Source: CAD feature listing. Evaluate the final solid. Frame: model axes, mm. Give positions to 0.01 mm unless a question says otherwise; leave off trailing zeros. Loops run counter-clockwise (first coordinate to the right, second up) from the corner with the lowest first, then second, coordinate; pieces in that order, holes last. Notation, with made-up numbers: M -27,73.5 L -8,73.5 A22 cw -8,87.5 Z; hole C 14,4 d6. An arc over 180 degrees is marked long. Answer in a Markdown table with one row per item.
```python
from build123d import *

# Parameters (mm, degrees)
EXTRUDE_1_DEPTH     = 3
EXTRUDE_2_DEPTH     = 200
FILLET_1_R          = 4
SKETCH_4_W          = 25
SKETCH_4_H          = 25
CUT_EXTRUDE_1_DEPTH = 4
FILLET_3_R          = 8
SKETCH_5_W          = 15
SKETCH_5_H          = 20
CUT_EXTRUDE_2_DEPTH = 10
FILLET_4_R          = 10
FILLET_5_R          = 10
SKETCH_7_R          = 1.05
SKETCH_7_R_2        = 1
CUT_EXTRUDE_3_DEPTH = 5


with BuildPart() as part:
    # 草图1 → 凸台-拉伸1 (new body)
    with BuildSketch(Plane.XY):
        Polygon((-68.534318099, 4.283164377), (-80.94435421, -20.816457208), (-55.844732625, -33.22649332), (-43.434696514, -8.126871734), align=None)
    extrude(amount=EXTRUDE_1_DEPTH)

    # 草图2 → 凸台-拉伸2 (add)
    with BuildSketch(Plane.XY.offset(3)):
        Polygon((-87.038364402, -64.656684429), (-38.284651107, 33.948971798), (-35.595405937, 32.619325071), (-84.349119232, -65.986331156), align=None)
    extrude(amount=EXTRUDE_2_DEPTH)

    # 圆角1
    fillet_1_edges = [part.edges().sort_by_distance(p)[0] for p in [
        (-59.529047009, -15.787087985, 3),
        (-62.218292179, -14.457441259, 3),
    ]]
    fillet(fillet_1_edges, radius=FILLET_1_R)

    # 草图4 → 切除-拉伸1 (cut)
    with BuildSketch(Plane(origin=(-44.25211262, 21.879625307, 0), x_dir=(0, 0, 1), z_dir=(-0.8964150566080468, 0.4432155754104229, 0))):
        with Locations((15.5, -84.035984194)):
            Rectangle(SKETCH_4_W, SKETCH_4_H)
    extrude(amount=-CUT_EXTRUDE_1_DEPTH, mode=Mode.SUBTRACT)

    # 圆角3
    fillet_3_edges = [part.edges().sort_by_distance(p)[0] for p in [
        (-74.613352432, -42.911131377, 3),
        (-74.613352432, -42.911131377, 28),
    ]]
    fillet(fillet_3_edges, radius=FILLET_3_R)

    # 草图5 → 切除-拉伸2 (cut)
    with BuildSketch(Plane(origin=(-41.56286745, 20.54997858, 0), x_dir=(0, 0, -1), z_dir=(0.8964150566080469, -0.4432155754104229, 0))):
        with Locations((-60.5, -11.535984194)):
            Rectangle(SKETCH_5_W, SKETCH_5_H)
        with Locations((-30.5, -11.535984194)):
            Rectangle(SKETCH_5_W, SKETCH_5_H)
        with Locations((-90.5, -11.535984194)):
            Rectangle(SKETCH_5_W, SKETCH_5_H)
        with Locations((-120.5, -11.535984194)):
            Rectangle(SKETCH_5_W, SKETCH_5_H)
        with Locations((-150.5, -11.535984194)):
            Rectangle(SKETCH_5_W, SKETCH_5_H)
        with Locations((-180.5, -11.535984194)):
            Rectangle(SKETCH_5_W, SKETCH_5_H)
        with Locations((-60.5, -41.535984194)):
            Rectangle(SKETCH_5_W, SKETCH_5_H)
        with Locations((-90.5, -41.535984194)):
            Rectangle(SKETCH_5_W, SKETCH_5_H)
        with Locations((-120.5, -41.535984194)):
            Rectangle(SKETCH_5_W, SKETCH_5_H)
        with Locations((-150.5, -41.535984194)):
            Rectangle(SKETCH_5_W, SKETCH_5_H)
        with Locations((-180.5, -41.535984194)):
            Rectangle(SKETCH_5_W, SKETCH_5_H)
        with Locations((-60.5, -71.535984194)):
            Rectangle(SKETCH_5_W, SKETCH_5_H)
        with Locations((-90.5, -71.535984194)):
            Rectangle(SKETCH_5_W, SKETCH_5_H)
        with Locations((-120.5, -71.535984194)):
            Rectangle(SKETCH_5_W, SKETCH_5_H)
        with Locations((-150.5, -71.535984194)):
            Rectangle(SKETCH_5_W, SKETCH_5_H)
        with Locations((-180.5, -71.535984194)):
            Rectangle(SKETCH_5_W, SKETCH_5_H)
        with Locations((-30.5, -41.535984194)):
            Rectangle(SKETCH_5_W, SKETCH_5_H)
    extrude(amount=-CUT_EXTRUDE_2_DEPTH, mode=Mode.SUBTRACT)

    # 圆角4
    fillet_4_edges = [part.edges().sort_by_distance(p)[0] for p in [
        (-36.940028522, 33.284148434, 203),
    ]]
    fillet(fillet_4_edges, radius=FILLET_4_R)

    # 圆角5
    fillet_5_edges = [part.edges().sort_by_distance(p)[0] for p in [
        (-36.940028522, 33.284148434, 3),
    ]]
    fillet(fillet_5_edges, radius=FILLET_5_R)

    # 草图7 → 切除-拉伸3 (cut)
    with BuildSketch(Plane(origin=(0, 0, 0), x_dir=(-1, 0, 0), z_dir=(0, 0, -1))):
        with Locations((48.793219042, -9.939669659)):
            Circle(SKETCH_7_R)
        with Locations((66.721520174, -1.075358151)):
            Circle(SKETCH_7_R)
        with Locations((71.153675928, -10.039508717)):
            Circle(SKETCH_7_R_2)
        with Locations((68.912638286, -11.147547656)):
            Circle(SKETCH_7_R_2)
        with Locations((75.585831682, -19.003659283)):
            Circle(SKETCH_7_R)
        with Locations((57.65753055, -27.867970791)):
            Circle(SKETCH_7_R)
        with Locations((53.225374796, -18.903820225)):
            Circle(SKETCH_7_R_2)
        with Locations((55.466412437, -17.795781287)):
            Circle(SKETCH_7_R_2)
    extrude(amount=-CUT_EXTRUDE_3_DEPTH, mode=Mode.SUBTRACT)


solid = part.part
```
1) Material intervals for L1, parallel to Z at x = -79.5, y = -21; L2, parallel to Y at x = -71, z = 127; L3, parallel to X at y = -17.5, z = 74, sorted ascending.
Reply:
| item | result |
|---|---|
| L1 | z = 0 to 3 |
| L2 | y = -33.54 to -32.22 |
| L3 | x = -63.72 to -60.38 |
2) Pin query (flat end, axial travel): pin 1 Ø3.5 at (x, y) = (-69, -33) entering from -Z; pin 2 Ø5 at (y, z) = (20.5, 23) entering from -X; pin 3 Ø8 at (x, y) = (-82.5, -55) entering from -Z. Return the tip coordinate at first contact, or that it passes through.
Reply:
| item | result |
|---|---|
| pin 1 | stops at z = 3 |
| pin 2 | stops at x = -46.17 |
| pin 3 | stops at z = 28 |
3) Pull-direction query (Z, two-part tool) for faces 1 (the cylindrical face through (-75.66, -45.08, 25.72)), 2 (the flat face through (-75, -43, 158)), 3 (the flat face through (-68, -10, 3)); classes: released by +Z, released by -Z, zero draft, split by the parting line, or undercut.
Reply:
| item | result |
|---|---|
| face 1 | released by -Z |
| face 2 | undercut |
| face 3 | released by +Z |
4) Section A-A, the plane z = 184. Return loops of the section in (x, y).
Reply:
| item | result |
|---|---|
| outline | M -87.04,-64.66 L -84.35,-65.99 L -77.7,-52.54 L -80.39,-51.21 Z; M -71.53,-33.28 L -68.84,-34.61 L -64.4,-25.65 L -67.09,-24.32 Z; M -58.23,-6.39 L -55.54,-7.72 L -51.11,1.24 L -53.8,2.57 Z; M -44.93,20.5 L -42.24,19.17 L -35.6,32.62 L -38.28,33.95 Z |
5) Section C-C, the plane z = 106. Return loops of the section in (x, y), then the cut area to 3 significant figures.
Reply:
| item | result |
|---|---|
| outline | M -87.04,-64.66 L -84.35,-65.99 L -35.6,32.62 L -38.28,33.95 Z |
| area | 330 mm² |
6) Section B-B, the plane y = 6.5. Return loops of the section in (x, z), then the cut area to 3 significant figures.
Reply:
| item | result |
|---|---|
| outline | M -51.86,3 L -48.51,3 L -48.51,23 L -51.86,23 Z; M -51.86,38 L -48.51,38 L -48.51,53 L -51.86,53 Z; M -51.86,68 L -48.51,68 L -48.51,83 L -51.86,83 Z; M -51.86,98 L -48.51,98 L -48.51,113 L -51.86,113 Z; M -51.86,128 L -48.51,128 L -48.51,143 L -51.86,143 Z; M -51.86,158 L -48.51,158 L -48.51,173 L -51.86,173 Z; M -51.86,188 L -48.51,188 L -48.51,203 L -51.86,203 Z |
| area | 368 mm² |
7) Section D-D, the plane y = -40. Count the separate pieces of the cut face and the enclosed holes in it, then the cut area to 3 significant figures.
Reply:
| item | result |
|---|---|
| separate pieces | 6 |
| enclosed holes | 0 |
| area | 413 mm² |
